The listing builds one solid part. Answer for the finished solid, in the listing's coordinates (mm). Coordinates: 2 decimals unless noted, no trailing zeros. Write each loop counter-clockwise with the first axis right and the second up, starting at its lowest first coordinate (ties: lowest second). Pieces come first, ordered by that corner, then holes.
(1) Given P1, Ø1.5, axis at x = 4, z = -0.5, coming from the -Y side, flat-ended and moving along its own axis, determine where the tip first touches the part or whether it passes through.
(2) The part is cut by section A-A on x = 1.75. Determine the outline of the cut face in (y, z).
(3) The part is cut by section B-B on y = 1.75. Determine the outline of the cut face in (x, z), plus the area to 3 significant figures.
(4) The part is cut by section C-C on z = 1.55. Determine the outline of the cut face in (x, y).
(5) For a pull along Z with two mould halves and no side action, classify faces 1 (the flat face through (6.6, 0, 0)), 2 (the flat face through (0.47, 0.31, -0.12)) as +Z half, -Z half, draft (parallel to the pull), parting line (faces both ways), or undercut.
(6) Straight lines are drawn through the part: line 1 (Z direction, x = 2.75, y = 0.4); line 2 (X direction, y = -1.05, z = -0.05); line 3 (X direction, y = 0.35, z = -1.55). For each, find the intervals that lie inside material, in ascending order.
(7) The part is cut by section D-D on x = 4.5. Determine the outline of the cut face in (y, z), plus the area to 3 significant figures.
from build123d import *

# Parameters (mm, degrees)
PATTERN_LINEAR_1_COUNT = 12
PATTERN_LINEAR_1_PITCH = 0.4


with BuildPart() as part:
    # 草图2 → Revolve 808 (revolve)
    with BuildSketch(Plane.XY, mode=Mode.PRIVATE) as revolve_808_sk:
        with BuildLine():
            Line((0, 0), (6.6, 0))
            Line((6.6, 0), (6.6, 1))
            Line((6.6, 1), (2.4, 1))
            Line((2.4, 1), (2.266, 0.866))
            Line((2.266, 0.866), (2.034, 0.866))
            ThreePointArc((2.034, 0.866), (1.727115657, 0.993115657), (1.6, 1.3))
            Line((1.6, 1.3), (1.6, 2))
            Line((1.6, 2), (1.459687576, 2))
            ThreePointArc((1.459687576, 2), (0.40373114, 1.23801129), (0, 0))
        make_face()
    revolve(revolve_808_sk.sketch.rotate(Axis((-1.331757704, 0, 0), (1, 0, 0)), 90), axis=Axis((-1.331757704, 0, 0), (1, 0, 0)))

    # 草图3 → 切除-旋转1 (revolve, cut)
    with BuildSketch(Plane.XY, mode=Mode.PRIVATE) as cut_revolve_1_sk:
        Polygon((6.402166402, 1), (6.802166402, 1), (6.6, 0.6536), align=None)
    cut_revolve_1 = revolve(cut_revolve_1_sk.sketch.rotate(Axis((-0.242766179, 0, 0), (1, 0, 0)), 90), axis=Axis((-0.242766179, 0, 0), (1, 0, 0)), mode=Mode.SUBTRACT)

    # 阵列(线性)1: 切除-旋转1 ×12
    with Locations(*[(-i * PATTERN_LINEAR_1_PITCH, 0, 0) for i in range(1, PATTERN_LINEAR_1_COUNT)]):
        add(cut_revolve_1, mode=Mode.SUBTRACT)

    # 草图5 → 切除-放样1 section 0
    with BuildSketch(Plane(origin=(0, 0, 0), x_dir=(0, 0, -1), z_dir=(1, 0, 0)), mode=Mode.PRIVATE) as loft_1_s0:
        with BuildLine():
            Line((0.2, 0.95), (-0.2, 0.95))
            Line((-0.2, 0.95), (-0.2, -0.95))
            Line((-0.2, -0.95), (0.2, -0.95))
            Line((0.2, -0.95), (0.2, 0.95))
        make_face()
    loft_1 = loft([Vertex(1.2, 0, 0), loft_1_s0.sketch], mode=Mode.SUBTRACT)

    # 镜向1: 切除-放样1 across plane
    add(loft_1.mirror(Plane(origin=(0, 0, 0), x_dir=(0, 0.7071067811865462, 0.7071067811865488), z_dir=(0, -0.7071067811865488, 0.7071067811865462))), mode=Mode.SUBTRACT)


solid = part.part
Model answer:
1. P1: stops at y = -1
2. outline: circle Ø1.94 at (0, 0)
3. outline: (1.46, -0.97) - (1.6, -0.97) - (1.6, 0.97) - (1.46, 0.97) arc R1.16 ccw to start
3. area: 0.981 mm2
4. outline: (1.46, -1.26) - (1.6, -1.26) - (1.6, 1.26) - (1.46, 1.26) arc R1.42 ccw to start
5. face 1: draft
5. face 2: undercut
6. line 1: z = -0.82 to 0.82
6. line 2: x = 0.28 to 1.68
6. line 3: x = 0.73 to 1.6
7. outline: circle Ø1.66 at (0, 0)
7. area: 2.16 mm2
